from build123d import *

# Parameters (mm, degrees)
BOSS_EXTRUDE1_DEPTH = 60
SKETCH4_R           = 3
CUT_EXTRUDE1_DEPTH  = 60
CHAMFER1_SIZE       = 5


with BuildPart() as part:
    # Sketch1 → Boss-Extrude1 (new body)
    with BuildSketch(Plane.XY):
        with BuildLine():
            Line((-10, 20), (10, 20))
            ThreePointArc((10, 20), (30, 0), (10, -20))
            Line((10, -20), (-10, -20))
            ThreePointArc((-10, -20), (-30, 0), (-10, 20))
        make_face()
        with BuildLine():
            Line((-7.5, 12.5), (7.5, 12.5))
            ThreePointArc((7.5, 12.5), (20, 0), (7.5, -12.5))
            Line((7.5, -12.5), (-7.5, -12.5))
            ThreePointArc((-7.5, -12.5), (-20, 0), (-7.5, 12.5))
        make_face(mode=Mode.SUBTRACT)
    extrude(amount=BOSS_EXTRUDE1_DEPTH)

    # Sketch4 → Cut-Extrude1 (cut)
    with BuildSketch(Plane.XZ.offset(20)):
        with Locations(Location((0, 32, 0), (0, 0, 270))):  # turned: the seam where the file's is
            Circle(SKETCH4_R)
    extrude(amount=-CUT_EXTRUDE1_DEPTH, mode=Mode.SUBTRACT)

    # Chamfer1
    chamfer1_edges = [part.edges().sort_by_distance(p)[0] for p in [
        (30, 0, 60),
        (0, 20, 60),
        (-30, 0, 60),
        (0, -20, 60),
    ]]
    chamfer(chamfer1_edges, length=CHAMFER1_SIZE)


solid = part.part
Here's how the part is built. I have some questions about the finished solid (model axes, mm). A direction names the side the tool comes from. Round coordinates to 2 decimals unless told otherwise and drop trailing zeros. Order: outer loops, then holes, each group sorted by start corner. A loop starts at its lowest first (then second) coordinate and runs counter-clockwise, first axis right, second up. Notation, with made-up numbers: (-9.5, 1.25) -> (-1.5, 1.25) arc R14 ccw to (-1.5, 13.25) -> close; hole circle Ø10 at (-6.75, 0.25). An arc over 180 degrees is marked (long way). Use CSV: the item, a comma, the result in double quotes.
1. I'm going to push flat-ended pins straight in: P1, Ø10, axis at x = -23, z = 31.5, coming from the -Y side; P2, Ø10, axis at x = -12.5, z = 28, coming from the -Y side; P3, Ø5.5, axis at x = 0, z = 32, coming from the -Y side; P4, Ø4, axis at x = -13, z = 50, coming from the +Y side (3 decimals). Where does each tip first touch, or does it pass through?
Recorded:
P1,"stops at y = -18.33"
P2,"stops at y = -20"
P3,"passes through"
P4,"stops at y = 19.975"
2. Which directions (+Z, -Z, +X, -X, +Y, -Y) give clear straight access to the entire face, cutting with the end or side of a thin tool? Please do faces 1 (the face through (20, 0, 30)), 2 (the face through (-30, 0, 27)).
Recorded:
face 1,"+Z, -Z"
face 2,"+Z, -Z, -X"
3. Thinking about a two-plate mould opening in Y: for faces 3 (the face through (-2, 13, 60)), 4 (the face through (3, -12.5, 30)), 5 (the face through (30, 0, 27)), which applies, pulls with the +Y half, pulls with the -Y half, needs draft (parallel to the pull), parting line crosses it, or undercut?
Recorded:
face 3,"needs draft"
face 4,"undercut"
face 5,"parting line crosses it"
4. I need wall thicknesses on line 1 along Y through (x, z) = (5, 55); line 2 along Y through (x, z) = (-16, 31.5); line 3 along X through (y, z) = (-16, 32). Which ranges of each line are inside material? Lowest first, please.
Recorded:
line 1,"y = -20 to -12.5, 12.5 to 20"
line 2,"y = -19.08 to -9.17, 9.17 to 19.08"
line 3,"x = -22 to -3, 3 to 22"
5. I want a section at D-D on z = 32. List the corners of the cut face in (x, y) for me, and give its area (3 significant figures).
Recorded:
outline,"(-10, -20) -> (-3, -20) -> (-3, -12.5) -> (-7.5, -12.5) arc R12.5 cw to (-7.5, 12.5) -> (-3, 12.5) -> (-3, 20) -> (-10, 20) arc R20 ccw to start; (3, -20) -> (10, -20) arc R20 ccw to (10, 20) -> (3, 20) -> (3, 12.5) -> (7.5, 12.5) arc R12.5 cw to (7.5, -12.5) -> (3, -12.5) -> close"
area,"1,100 mm2"
6. I want a section at A-A on z = 50.5. List the corners of the cut face in (x, y) for me.
Recorded:
outline,"(-10, -20) -> (10, -20) arc R20 ccw to (10, 20) -> (-10, 20) arc R20 ccw to start; hole (-7.5, -12.5) -> (7.5, -12.5) arc R12.5 ccw to (7.5, 12.5) -> (-7.5, 12.5) arc R12.5 ccw to start"
7. I want a section at C-C on x = 0. List the corners of the cut face in (y, z) for me, and give its area (3 significant figures).
Recorded:
outline,"(-20, 0) -> (-12.5, 0) -> (-12.5, 29) -> (-20, 29) -> close; (-20, 35) -> (-12.5, 35) -> (-12.5, 60) -> (-15, 60) -> (-20, 55) -> close; (12.5, 0) -> (20, 0) -> (20, 29) -> (12.5, 29) -> close; (12.5, 35) -> (20, 35) -> (20, 55) -> (15, 60) -> (12.5, 60) -> close"
area,"785 mm2"
8. I want a section at B-B on y = 0. List the corners of the cut face in (x, z) for me.
Recorded:
outline,"(-30, 0) -> (-20, 0) -> (-20, 60) -> (-25, 60) -> (-30, 55) -> close; (20, 0) -> (30, 0) -> (30, 55) -> (25, 60) -> (20, 60) -> close"
